Read the model definition and answer for the solid it produces. Units are mm, in the model's axes. Face numbers are marked on the shaded views. A direction names the side the tool comes from. Give positions to 0.01 mm unless a question says otherwise; leave off trailing zeros. Order: outer loops, then holes, each group sorted by start corner. A loop starts at its lowest first (then second) coordinate and runs counter-clockwise, first axis right, second up. Notation, with made-up numbers: (-29, -25) - (-7, -25) arc R31 ccw to (-7, 13) - close; hole circle Ø2 at (-33.75, 11.5). An arc over 180 degrees is marked (long way). Answer as CSV lines item,"result". Start each with the question number.
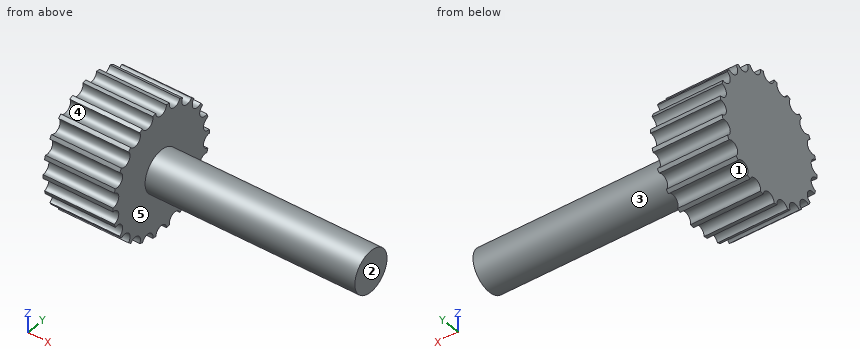
from build123d import *

# Parameters (mm, degrees)
SKETCH1_R           = 4.5
BOSS_EXTRUDE1_DEPTH = 5
SKETCH2_R           = 1.5
BOSS_EXTRUDE2_DEPTH = 20
SKETCH3_R           = 0.5
CUT_EXTRUDE2_DEPTH  = 5
CIRPATTERN1_COUNT   = 22


with BuildPart() as part:
    # Sketch1 → Boss-Extrude1 (new body)
    with BuildSketch(Plane(origin=(0, 0, 0), x_dir=(0, 0, -1), z_dir=(1, 0, 0))):
        Circle(SKETCH1_R)
    extrude(amount=BOSS_EXTRUDE1_DEPTH)

    # Sketch2 → Boss-Extrude2 (add)
    with BuildSketch(Plane(origin=(0, 0, 0), x_dir=(0, 0, -1), z_dir=(1, 0, 0))):
        Circle(SKETCH2_R)
    extrude(amount=BOSS_EXTRUDE2_DEPTH)

    # Sketch3 → Cut-Extrude2 (cut, symmetric)
    with BuildSketch(Plane(origin=(0, 0, 0), x_dir=(0, 0, -1), z_dir=(1, 0, 0))):
        with Locations((4.5, 0)):
            Circle(SKETCH3_R)
    cut_extrude2 = extrude(amount=CUT_EXTRUDE2_DEPTH, both=True, mode=Mode.SUBTRACT)

    # CirPattern1: Cut-Extrude2 ×22 about axis
    cirpattern1_axis = Axis((0, 0, 0), (1, 0, 0))
    for i in range(1, CIRPATTERN1_COUNT):
        add(cut_extrude2.rotate(cirpattern1_axis, i * 360 / CIRPATTERN1_COUNT), mode=Mode.SUBTRACT)


solid = part.part
(1) Section B-B, the plane z = -0.5 is taken. Write down the section's boundary in (x, y), and give its area (3 significant figures).
(2) Determine the mould class of the marked faces 1, 2 and 3 for opening direction Y: released by +Y, released by -Y, zero draft, split by the parting line, or undercut.
(3) Section D-D, the plane z = 3 is taken. Write down the section's boundary in (x, y), and give its area (3 significant figures).
(4) Section A-A, the plane y = 0 is taken. Write down the section's boundary in (x, z), and give its area (3 significant figures).
(5) Straight lines are drawn through the part: line 1 (Z direction, x = 12, y = 0); line 2 (X direction, y = 1.25, z = -2.75); line 3 (Z direction, x = 18.25, y = 1). For each, find the intervals that lie inside material, in ascending order. Write a range as [from, to].
(6) A flat-ended cylindrical pin translates along its axis: pin 1 Ø3 at (x, z) = (8, 1.5) entering from -Y. Find the tip coordinate at first contact, or state that the pin passes through.
(7) Section C-C, the plane x = 14.5 is taken. Write down the section's boundary in (y, z), and give its area (3 significant figures).
(8) Which of the six approach directions +Z, -Z, +X, -X, +Y, -Y give full straight-line access (tool end or side, diameter ignored) to the marked faces 4 and 5?
Checks:
1,outline,"(0, -3.97) - (5, -3.97) - (5, -1.41) - (20, -1.41) - (20, 1.41) - (5, 1.41) - (5, 3.97) - (0, 3.97) - close"
1,area,"82.2 mm²"
2,face 1,"undercut"
2,face 2,"zero draft"
2,face 3,"split by the parting line"
3,outline,"(0, -2.9) - (5, -2.9) - (5, 2.9) - (0, 2.9) - close"
3,area,"29.0 mm²"
4,outline,"(0, -4) - (5, -4) - (5, -1.5) - (20, -1.5) - (20, 1.5) - (5, 1.5) - (5, 4) - (0, 4) - close"
4,area,"85.0 mm²"
5,line 1,"z = [-1.5, 1.5]"
5,line 2,"x = [0, 5]"
5,line 3,"z = [-1.12, 1.12]"
6,pin 1,"stops at y = -1.5"
7,outline,"circle Ø3 at (0, 0)"
7,area,"7.07 mm²"
8,face 4,"+X, -X"
8,face 5,"+X"
